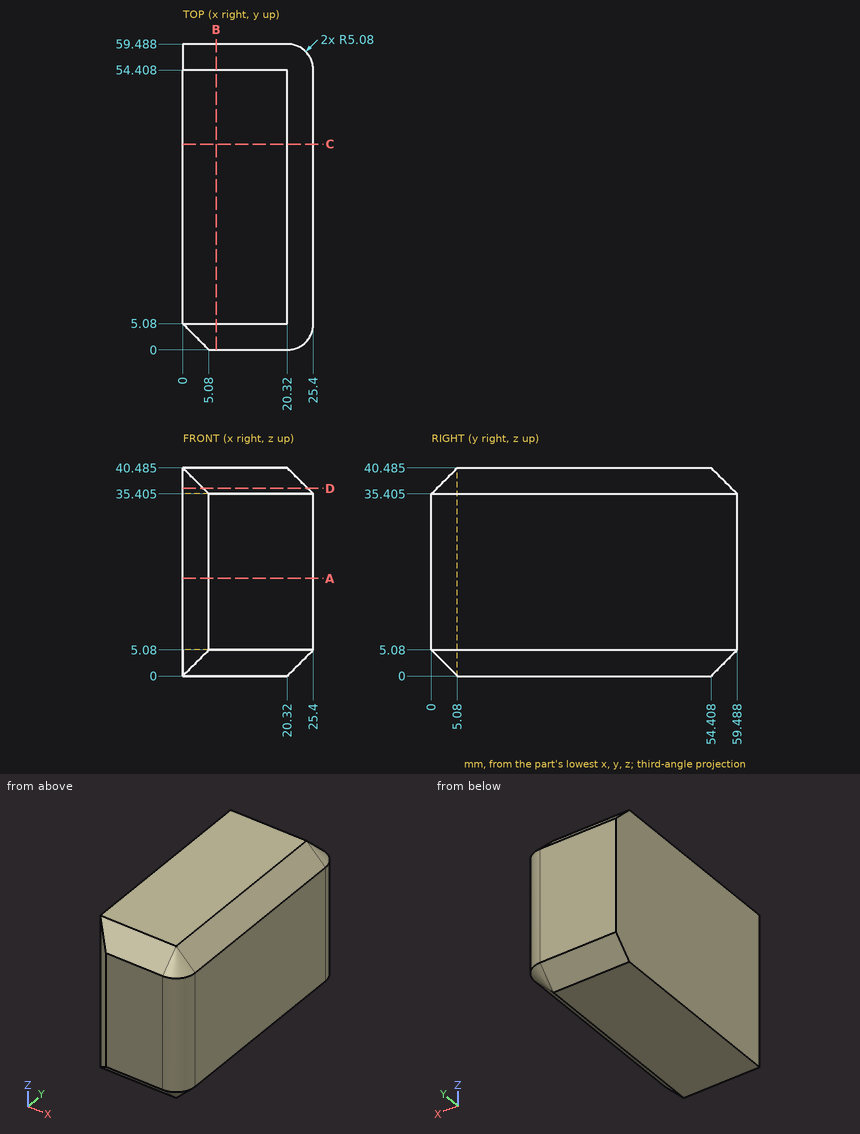
Design review of the part shown in the three views and the two pictorial views. Dimensions are in mm from the part's minimum x, y and z. Coordinates: 2 decimals unless noted, no trailing zeros. Loops run counter-clockwise (first coordinate to the right, second up) from the corner with the lowest first, then second, coordinate; pieces in that order, holes last. Notation, with made-up numbers: M 29,39 L 42,39 A19 ccw 42,59 Z; hole C 48,-3.5 d10. An arc over 180 degrees is marked long. One line per question, with ' | ' between items.
(1) Wall thickness on probe 1 along Y at (x, z) = (5, 10); probe 2 along Y at (x, z) = (21, 36); probe 3 along X at (y, z) = (26, 38.5) (1 decimal): over which ranges is each line inside the solid? List them lowest first.
Filled in:
probe 1: y = 0.08 to 59.49 | probe 2: y = 0.65 to 58.84 | probe 3: x = 0 to 22.3
(2) We need section C-C (y = 40). Give the boundary of the cut face in (x, z) (1 decimal), and give its area (3 significant figures).
Filled in:
outline: M 0,0 L 20.3,0 L 25.4,5.1 L 25.4,35.4 L 20.3,40.5 L 0,40.5 Z | area: 1,000 mm^2
(3) We need section D-D (z = 36.5). Give the boundary of the cut face in (x, y) (1 decimal).
Filled in:
outline: M 0,5.1 L 4,1.1 L 20.3,1.1 A4 ccw 24.3,5.1 L 24.3,54.4 A4 ccw 20.3,58.4 L 0,58.4 Z
(4) For pin 1 Ø1 at (x, y) = (21.5, 48) entering from +Z (1 decimal); pin 2 Ø2 at (x, z) = (22.5, 10) entering from -Y, all flat-tipped, find the tip position at first contact; note any pin that passes through.
Filled in:
pin 1: stops at z = 39.8 | pin 2: stops at y = 0.14
(5) We need section B-B (x = 6.5). Give the boundary of the cut face in (y, z) (1 decimal).
Filled in:
outline: M 0,5.1 L 5.1,0 L 54.4,0 L 59.5,5.1 L 59.5,35.4 L 54.4,40.5 L 5.1,40.5 L 0,35.4 Z
(6) We need section A-A (z = 19). Give the boundary of the cut face in (x, y).
Filled in:
outline: M 0,5.08 L 5.08,0 L 20.32,0 A5.08 ccw 25.4,5.08 L 25.4,54.41 A5.08 ccw 20.32,59.49 L 0,59.49 Z
